Geometry check sheet. Reference: drawing and pictorial views, mm from the part's lowest x, y, z. Coordinates: 2 decimals unless noted, no trailing zeros. Write each loop counter-clockwise with the first axis right and the second up, starting at its lowest first coordinate (ties: lowest second). Pieces come first, ordered by that corner, then holes. Notation, with made-up numbers: (74.25, 38.25) -> (115.25, 38.25) arc R12 cw to (115.25, 57.25) -> close; hole circle Ø3 at (-38, -24.5). An arc over 180 degrees is marked (long way). Use a Markdown table: item, result.
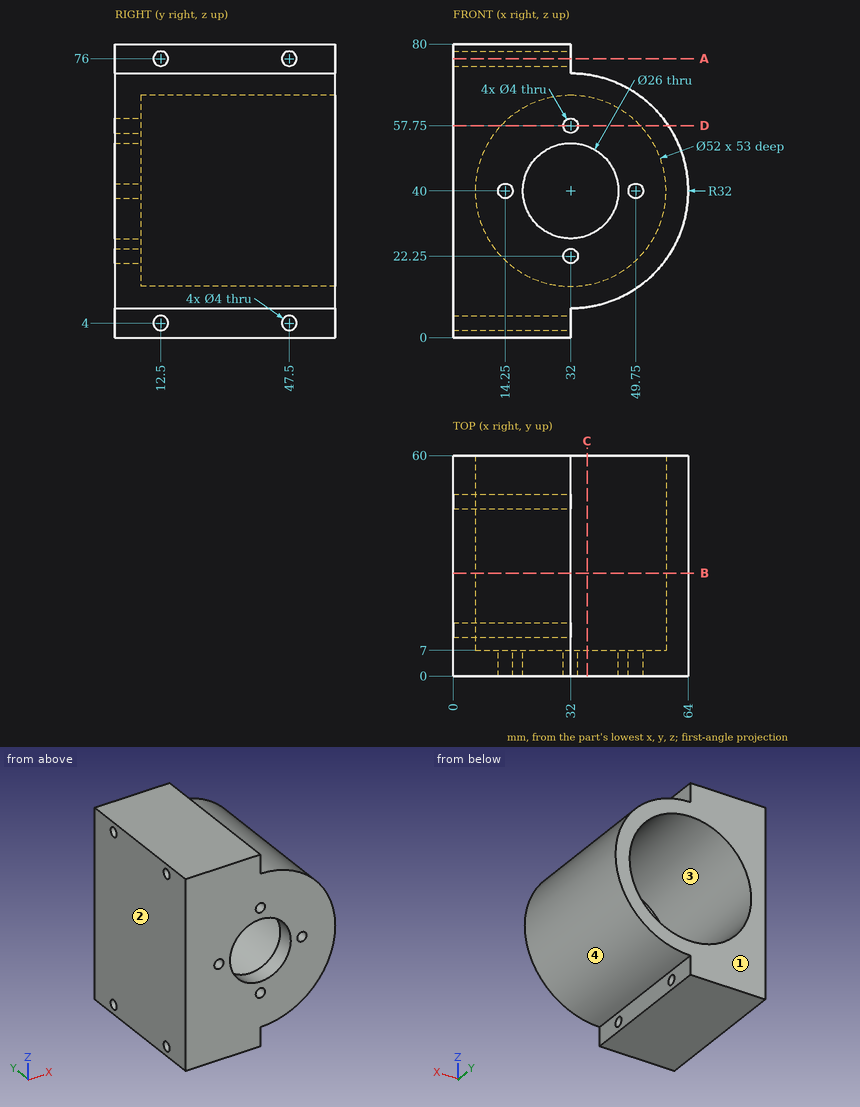
Item 1: Mould release check, pull along X, two halves, no side actions. Record for the marked faces 1, 2, 3 and 4: +X half, -X half, draft (parallel to the pull), parting line (faces both ways), or undercut.
Answer block:
| item | result |
|---|---|
| face 1 | draft |
| face 2 | -X half |
| face 3 | undercut |
| face 4 | +X half |
Item 2: Thickness scan on L1, parallel to X at y = 4.5, z = 40; L2, parallel to Z at x = 14.25, y = 1.5; L3, parallel to Z at x = 32.5, y = 5. Record the ranges inside material, lowest first. Write a range as [from, to].
Answer block:
| item | result |
|---|---|
| L1 | x = [0, 12.25], [16.25, 19], [45, 47.75], [51.75, 64] |
| L2 | z = [0, 38], [42, 80] |
| L3 | z = [8, 20.31], [24.19, 27.01], [52.99, 55.81], [59.69, 72] |
Item 3: Section check C-C on x = 36.5. Record the boundary of the cut face in (y, z), then the cut area to 3 significant figures.
Answer block:
| item | result |
|---|---|
| outline | (0, 8.32) -> (60, 8.32) -> (60, 14.39) -> (7, 14.39) -> (7, 27.8) -> (0, 27.8) -> close; (0, 52.2) -> (7, 52.2) -> (7, 65.61) -> (60, 65.61) -> (60, 71.68) -> (0, 71.68) -> close |
| area | 917 mm^2 |
Item 4: Section check A-A on z = 76. Record the boundary of the cut face in (x, y), then the cut area to 3 significant figures.
Answer block:
| item | result |
|---|---|
| outline | (0, 0) -> (32, 0) -> (32, 10.5) -> (0, 10.5) -> close; (0, 14.5) -> (32, 14.5) -> (32, 45.5) -> (0, 45.5) -> close; (0, 49.5) -> (32, 49.5) -> (32, 60) -> (0, 60) -> close |
| area | 1,660 mm^2 |
Item 5: Depth check by flat-ended pin: P1, Ø4, axis at y = 16, z = 61, coming from the +X side; P2, Ø12, axis at x = 14, z = 33, coming from the +Y side; P3, Ø2.5, axis at y = 27.5, z = 5.5, coming from the +X side. Enter the tip coordinate at first touch or a pass-through.
Answer block:
| item | result |
|---|---|
| P1 | stops at x = 57.75 |
| P2 | stops at y = 7 |
| P3 | stops at x = 32 |
Item 6: Section check B-B on y = 28. Record the boundary of the cut face in (x, z).
Answer block:
| item | result |
|---|---|
| outline | (0, 0) -> (32, 0) -> (32, 8) arc R32 ccw to (32, 72) -> (32, 80) -> (0, 80) -> close; hole circle Ø52 at (32, 40) |
Item 7: Section check D-D on z = 57.75. Record the boundary of the cut face in (x, y).
Answer block:
| item | result |
|---|---|
| outline | (0, 0) -> (30, 0) -> (30, 7) -> (13, 7) -> (13, 60) -> (0, 60) -> close; (34, 0) -> (58.63, 0) -> (58.63, 60) -> (51, 60) -> (51, 7) -> (34, 7) -> close |
